Autodesk Inventor part; units mm, degrees
ref_plane "YZ Plane" through (0, 0, 0) normal (1, 0, 0) x (0, 1, 0)
ref_plane "XZ Plane" through (0, 0, 0) normal (0, 1, 0) x (-1, 0, 0)
ref_plane "XY Plane" through (0, 0, 0) normal (0, 0, 1) x (1, 0, 0)
sketch "Эскиз1" plane through (0, 0, 0) normal (0, 0, 1) x (1, 0, 0)
  circle A0 centre (0, 0) radius 7.95
  circle A1 centre (0, 0) radius 11
  circle A2 centre (0, 0) radius 6
  dimension "d0" = 15.9
  dimension "d1" = 22
  dimension "d2" = 12
extrude "Выдавливание1" add sketch "Эскиз1" against normal blind 2.5 contours A0
extrude "Выдавливание2" add sketch "Эскиз1" along normal blind 5 contours A0 | A1
sketch "Эскиз2" plane through (0, 0, 0) normal (0, 0, -1) x (-1, 0, 0)
  circle A0 centre (3.6709, -8.2173) radius 1.5
  circle A1 centre (-3.6709, 8.2173) radius 1.5
  circle A2 centre (3.6709, -8.2173) radius 1.5
  circle A3 centre (-3.6709, 8.2173) radius 1.5
  point P0 (0, 0)
  dimension "d7" = 3
  dimension "d8" = 3
extrude "Выдавливание3" cut sketch "Эскиз2" along normal mid plane 30
properties part number "MELLOW barrier adapter"
Verification items for the finished model (mm, model axes). A direction names the side the tool comes from. Give positions to 0.01 mm unless a question says otherwise; leave off trailing zeros. Order: outer loops, then holes, each group sorted by start corner. A loop starts at its lowest first (then second) coordinate and runs counter-clockwise, first axis right, second up. Notation, with made-up numbers: M 26.5,60.5 L 66.5,60.5 A26 cw 66.5,92.5 Z; hole C 48,78 d2. An arc over 180 degrees is marked long. Answer in a Markdown table with one row per item. Add a question column.
Item 1: Mould release check, pull along X, two halves, no side actions. Record for faces 1 (the flat face through (-2, 6, -2.5)), 2 (the cylindrical face through (3.87, 6.73, 2.14)), 3 (the cylindrical face through (-2.38, 10.74, 2.46)): released by +X, released by -X, zero draft, split by the parting line, or undercut.
Item 2: Section check A-A, the plane y = 0. Enter the section's corners in (x, z).
Item 3: Gauge pin test, flat ends, axial feed: pin 1 (4 mm diameter, centred on x = -4, z = 3, fed in from +Y); pin 2 (4 mm diameter, centred on y = -6.5, z = 3, fed in from -X); pin 3 (1 mm diameter, centred on y = -5.5, z = 2, fed in from +X). Record the tip position at first contact, or that the pin passes through.
Item 4: Scan lines: probe 1 along Y at (x, z) = (-2.5, 0.25); probe 2 along Y at (x, z) = (4.75, 0.25); probe 3 along Z at (x, y) = (1.5, -9.5). Record each from-to range of solid material in increasing order. Write a range as from..to.
Item 5: Section check D-D, the plane y = -9. Enter the section's corners in (x, z).
Item 6: Section check C-C, the plane z = -1. Enter the section's corners in (x, y), and give its area (3 significant figures).
Item 7: Tool access check on faces 4 (the flat face through (5, -5, 5)), 5 (the flat face through (8.1, 0.1, 0)). Record the directions out of +Z, -Z, +X, -X, +Y, -Y that give a thin tool (end or side, any length) a straight path to the whole face; none if there is none.
Filled sheet:
| question | item | result |
|---|---|---|
| 1 | face 1 | zero draft |
| 1 | face 2 | undercut |
| 1 | face 3 | split by the parting line |
| 2 | outline | M -11,0 L -7.95,0 L -7.95,-2.5 L -6,-2.5 L -6,5 L -11,5 Z; M 6,-2.5 L 7.95,-2.5 L 7.95,0 L 11,0 L 11,5 L 6,5 Z |
| 3 | pin 1 | stops at y = 10.82 |
| 3 | pin 2 | stops at x = -10.04 |
| 3 | pin 3 | stops at x = 9.8 |
| 4 | probe 1 | y = -10.71..-9.15, -7.28..-5.45, 5.45..10.71 |
| 4 | probe 2 | y = -9.92..-3.67, 3.67..7.18, 9.26..9.92 |
| 4 | probe 3 | z = 0..5 |
| 5 | outline | M -6.32,0 L -4.95,0 L -4.95,5 L -6.32,5 Z; M -2.39,0 L 6.32,0 L 6.32,5 L -2.39,5 Z |
| 6 | outline | M -4.13,-6.79 A1.5 cw -2.3,-7.61 A7.95 ccw 4.13,6.79 A1.5 cw 2.3,7.61 A7.95 ccw Z; hole C 0,0 d12 |
| 6 | area | 84.2 mm^2 |
| 7 | face 4 | +Z, +X, -X, +Y, -Y |
| 7 | face 5 | -Z |
